For this review, take the finished solid that the model builds, in its own axes (mm). Coordinates: 2 decimals unless noted, no trailing zeros. Write each loop counter-clockwise with the first axis right and the second up, starting at its lowest first coordinate (ties: lowest second). Pieces come first, ordered by that corner, then holes.
Solid Edge part; units mm, degrees
sketch "Sketch1" plane through (0, 0, 0) normal (0, 0, 1) x (1, 0, 0)
  circle A0 centre (0, 0) radius 4.25
extrude "Protrusion1" add sketch "Sketch1" along normal blind 5
sketch "Sketch2" plane through (0, 0, 0) normal (0, 0, -1) x (1, 0, 0)
  circle A0 centre (0, 0) radius 2.5
extrude "Protrusion2" add sketch "Sketch2" along normal blind 100
sketch "Sketch3" plane through (0, 0, -100) normal (0, 0, -1) x (1, 0, 0)
  circle A0 centre (0, 0) radius 2.4997
extrude "Cutout1" cut sketch "Sketch3" against normal blind 22 flip side to cut
chamfer "Chamfer_1" distance 0.375 angle 45 1 edges at (-2.4997, 0, -100)
sketch "Sketch4" plane through (0, 0, 5) normal (0, 0, 1) x (1, 0, 0)
  line L0 (-1.1547, 2) -> (1.1547, 2)
  line L1 (2.3094, 0) -> (1.1547, 2)
  line L2 (1.1547, -2) -> (2.3094, 0)
  line L3 (-1.1547, -2) -> (1.1547, -2)
  line L4 (-2.3094, 0) -> (-1.1547, -2)
  line L5 (-1.1547, 2) -> (-2.3094, 0)
extrude "Cutout2" cut sketch "Sketch4" against normal blind 2.5
properties part number "170766" material "Stainless Steel, 304"
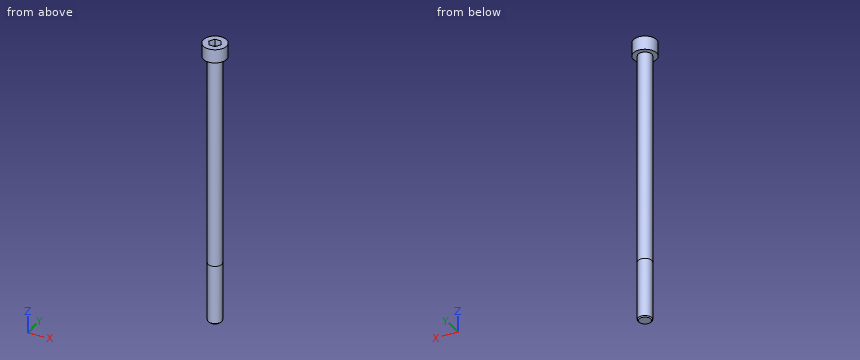
Q1. Add section B-B (z = -36.5). State the section outline as (x, y) points, then the cut area to 3 significant figures.
Ans:
outline: circle Ø5 at (0, 0)
area: 19.6 mm2
Q2. For probe 1 along Z at (x, y) = (2, 0.75); probe 2 along Z at (x, y) = (-2, 1.75); probe 3 along Y at (x, z) = (1.5, -28), list the stretches that pass through material, from the lowest coordinate up.
Ans:
probe 1: z = -99.99 to 5
probe 2: z = 0 to 5
probe 3: y = -2 to 2
Q3. Clearance check with flat-ended pins moving along their axes: pin 1 Ø3 at (y, z) = (1.5, -24.5) entering from +X; pin 2 Ø1.2 at (x, z) = (0.5, 4.5) entering from -Y; pin 3 Ø3 at (x, z) = (0.5, -8.5) entering from +Y. State where each tip first meets the part, or that it passes through.
Ans:
pin 1: stops at x = 2.5
pin 2: stops at y = -4.25
pin 3: stops at y = 2.5
